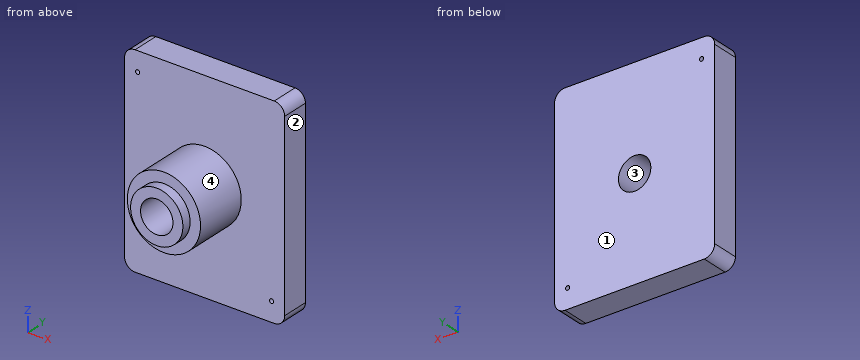
```python
from build123d import *

# Parameters (mm, degrees)
F0_W      = 76.5
F0_H      = 96.5
F1_DEPTH  = 13
F2_R      = 17.5
F3_DEPTH  = 30
F4_R      = 5
F5_R      = 17.5
F5_R_2    = 12.5
F6_DEPTH  = 4.5
F7_R      = 7.75
F8_DEPTH  = 43
F9_R      = 1
F10_DEPTH = 13


with BuildPart() as f1:
    # F0 (on Front) → F1 (new body)
    with BuildSketch(Plane.XZ):
        with Locations((38.25, 48.25)):
            Rectangle(F0_W, F0_H)
    extrude(amount=F1_DEPTH)

    # F2 (on face) → F3 (join)
    with BuildSketch(Plane.XZ.offset(13)):
        with Locations((38.25, 48.25)):
            Circle(F2_R)
    extrude(amount=F3_DEPTH)

    # F4
    f4_edges = [f1.edges().sort_by_distance(p)[0] for p in [
        (76.5, -6.5, 96.5),
        (0, -6.5, 96.5),
        (0, -6.5, 0),
        (76.5, -6.5, 0),
    ]]
    fillet(f4_edges, radius=F4_R)

    # F5 (on face) → F6 (cut)
    with BuildSketch(Plane.XZ.offset(43)):
        with Locations((38.25, 48.25)):
            Circle(F5_R)
        with Locations((38.25, 48.25)):
            Circle(F5_R_2, mode=Mode.SUBTRACT)
    extrude(amount=-F6_DEPTH, mode=Mode.SUBTRACT)

    # F7 (on face) → F8 (cut, through all)
    with BuildSketch(Plane.XZ.offset(43)):
        with Locations((38.25, 48.25)):
            Circle(F7_R)
    extrude(amount=-F8_DEPTH, mode=Mode.SUBTRACT)

    # F9 (on face) → F10 (cut, through all)
    with BuildSketch(Plane.XZ.offset(13)):
        with Locations((6.25, 87.25)):
            Circle(F9_R)
        with Locations((70.25, 9.25)):
            Circle(F9_R)
    extrude(amount=-F10_DEPTH, mode=Mode.SUBTRACT)


solid = f1.part
```
Model file for the job. Use its own axes, mm. Face numbers are marked on the shaded views. Coordinates: 2 decimals unless noted, no trailing zeros. Loops run counter-clockwise (first coordinate to the right, second up) from the corner with the lowest first, then second, coordinate; pieces in that order, holes last. Notation, with made-up numbers: (68, 69.5) - (125, 69.5) arc R22 cw to (125, 108.5) - close; hole circle Ø1 at (-35.75, 50). An arc over 180 degrees is marked (long way). Write item = value, one per line. Start each with the question number.
Item 1: Saw through at B-B, the plane y = -8.5. List the corners of the cut face in (x, z), then the cut area to 3 significant figures.
Item 2: Saw through at C-C, the plane z = 48.25. List the corners of the cut face in (x, y).
Item 3: Pull direction X, two halves, no side cores. Call the marked faces 1, 2, 3 and 4: +X half, -X half, draft (parallel to the pull), parting line (faces both ways), or undercut.
Item 4: Saw through at A-A, the plane x = 38.25. List the corners of the cut face in (y, z).
Item 5: Saw through at D-D, the plane y = -24. List the corners of the cut face in (x, z).
Item 6: Wall check: probe 1 along X at (y, z) = (-4.5, 48.5); probe 2 along X at (y, z) = (-19, 48); probe 3 along Z at (x, y) = (6.25, -3.5). Give the ranges that are in metal, low to high. Write a range as [from, to].
Item 7: Drop flat-ended pins along their axis: pin 1 Ø12 at (y, z) = (-29, 36.5) entering from -X; pin 2 Ø3 at (x, y) = (29, -27) entering from -Z; pin 3 Ø12 at (x, z) = (62.5, 60) entering from -Y. Give the stop position or say it passes through.
Answers:
q1.outline = (0, 5) arc R5 ccw to (5, 0) - (71.5, 0) arc R5 ccw to (76.5, 5) - (76.5, 91.5) arc R5 ccw to (71.5, 96.5) - (5, 96.5) arc R5 ccw to (0, 91.5) - close; hole circle Ø2 at (6.25, 87.25); hole circle Ø15.5 at (38.25, 48.25); hole circle Ø2 at (70.25, 9.25)
q1.area = 7,170 mm2
q2.outline = (0, -13) - (20.75, -13) - (20.75, -38.5) - (25.75, -38.5) - (25.75, -43) - (30.5, -43) - (30.5, 0) - (0, 0) - close; (46, -43) - (50.75, -43) - (50.75, -38.5) - (55.75, -38.5) - (55.75, -13) - (76.5, -13) - (76.5, 0) - (46, 0) - close
q3.face_1 = draft
q3.face_2 = +X half
q3.face_3 = undercut
q3.face_4 = parting line
q4.outline = (-43, 35.75) - (-38.5, 35.75) - (-38.5, 30.75) - (-13, 30.75) - (-13, 0) - (0, 0) - (0, 40.5) - (-43, 40.5) - close; (-43, 56) - (0, 56) - (0, 96.5) - (-13, 96.5) - (-13, 65.75) - (-38.5, 65.75) - (-38.5, 60.75) - (-43, 60.75) - close
q5.outline = circle Ø35 at (38.25, 48.25); hole circle Ø15.5 at (38.25, 48.25)
q6.probe_1 = [0, 30.5], [46, 76.5]
q6.probe_2 = [20.75, 30.5], [46, 55.75]
q6.probe_3 = [0, 86.25], [88.25, 96.5]
q7.pin_1 = 21.72
q7.pin_2 = 32.56
q7.pin_3 = -13
